from build123d import *

# Parameters (mm, degrees)
F0_R     = 8.25
F1_DEPTH = 10
F2_SIZE  = 6
F3_T     = -0.8
F4_R     = 1.75
F5_DEPTH = 25
F6_R     = 8.25
F6_R_2   = 3.75
F7_DEPTH = 2


with BuildPart() as f1:
    # F0 (on Top) → F1 (new body)
    with BuildSketch(Plane.XY):
        Circle(F0_R)
    extrude(amount=F1_DEPTH)

    # F2
    f2_edges = [f1.edges().sort_by_distance(p)[0] for p in [
        (-8.25, 0, 10),
    ]]
    chamfer(f2_edges, length=F2_SIZE)

    # F3
    f3_openings = [f1.faces().sort_by_distance(p)[0] for p in [
        (0, 0, 0),
    ]]
    offset(amount=F3_T, openings=f3_openings)

    # F4 (on face) → F5 (cut)
    with BuildSketch(Plane.XY.offset(10)):
        Circle(F4_R)
    extrude(amount=-F5_DEPTH, mode=Mode.SUBTRACT)

    # F6 (on Top) → F7 (join)
    with BuildSketch(Plane.XY):
        Circle(F6_R)
        Circle(F6_R_2, mode=Mode.SUBTRACT)
    extrude(amount=-F7_DEPTH)


solid = f1.part
Build history of the part. All positions in model axes, mm. A direction names the side the tool comes from. Coordinates: 2 decimals unless noted, no trailing zeros. Write each loop counter-clockwise with the first axis right and the second up, starting at its lowest first coordinate (ties: lowest second). Pieces come first, ordered by that corner, then holes.
(1) Cut at D-D on z = -1. List the corners of the cut face in (x, y).
(2) Cut at A-A on y = 0. List the corners of the cut face in (x, z), and give its area (3 significant figures).
(3) Pin check, flat tips, straight feed: pin 1 Ø1.5 at (y, z) = (2.5, 6.5) entering from +X; pin 2 Ø3 at (x, y) = (1, 1) entering from -Z; pin 3 Ø2 at (x, y) = (0, 0) entering from +Z; pin 4 Ø2 at (y, z) = (-4.5, 0) entering from +X. Stop position of each tip, or through.
(4) Drill centre lines: line 1 (Y direction, x = 0, z = 2.55); line 2 (Y direction, x = 0, z = -1.3); line 3 (X direction, y = -2, z = 5.75). Where is each one in solid material? Low to high.
(5) 3-axis set-ups, long thin cutter, end or side, ignore diameter. For faces 1 (the cylindrical face through (-3.746, 0.165, -0.986)), 2 (the conical face through (-0.47, -2.14, 8.93)), 3 (the flat face through (0, -2, 10)): which of +Z, -Z, +X, -X, +Y, -Y reach the whole face in a straight line?
(6) Cut at C-C on z = 0.5. List the corners of the cut face in (x, y).
(7) Mould opens along Y. For faces 4 (the cylindrical face through (7.62, -3.16, 1.04)), 5 (the flat face through (2, -4, -2)), 6 (the flat face through (3, -3, 0)) say: pulls with the +Y half, pulls with the -Y half, needs draft (parallel to the pull), parting line crosses it, or undercut.
Working result:
1. outline: circle Ø16.5 at (0, 0); hole circle Ø7.5 at (0, 0)
2. outline: (-8.25, -2) - (-3.75, -2) - (-3.75, 0) - (-7.45, 0) - (-7.45, 3.67) - (-1.92, 9.2) - (-1.75, 9.2) - (-1.75, 10) - (-2.25, 10) - (-8.25, 4) - close; (1.75, 9.2) - (1.92, 9.2) - (7.45, 3.67) - (7.45, 0) - (3.75, 0) - (3.75, -2) - (8.25, -2) - (8.25, 4) - (2.25, 10) - (1.75, 10) - close
2. area: 37.7 mm2
3. pin 1: stops at x = 6.05
3. pin 2: stops at z = 8.2
3. pin 3: passes through
3. pin 4: stops at x = 7.47
4. line 1: y = -8.25 to -7.45, 7.45 to 8.25
4. line 2: y = -8.25 to -3.75, 3.75 to 8.25
4. line 3: x = -6.18 to -4.98, 4.98 to 6.18
5. face 1: -Z
5. face 2: none
5. face 3: +Z, +X, -X, +Y, -Y
6. outline: circle Ø16.5 at (0, 0); hole circle Ø14.9 at (0, 0)
7. face 4: parting line crosses it
7. face 5: needs draft
7. face 6: undercut
